```python
from build123d import *

# Parameters (mm, degrees)
SKETCH_W        = 19.05
SKETCH_H        = 9.525
PAD_DEPTH       = 215.9
SKETCH001_W     = 9.525
SKETCH001_H     = 2.38125
POCKET_DEPTH    = 215.901
SKETCH002_W     = 14.2875
SKETCH002_H     = 3.175
POCKET001_DEPTH = 215.901
SKETCH003_W     = 11.1125
SKETCH003_H     = 1.5875
POCKET002_DEPTH = 215.901


with BuildPart() as part:
    # Sketch → Pad (new body)
    with BuildSketch(Plane.XZ):
        Rectangle(SKETCH_W, SKETCH_H)
    extrude(amount=PAD_DEPTH)

    # Sketch001 (on Face6 of Pad) → Pocket (cut, through all)
    with BuildSketch(Plane.XZ.offset(215.9)):
        with Locations((0, 3.571875)):
            Rectangle(SKETCH001_W, SKETCH001_H)
    extrude(amount=-POCKET_DEPTH, mode=Mode.SUBTRACT)

    # Sketch002 (on Face5 of Pocket) → Pocket001 (cut, through all)
    with BuildSketch(Plane.XZ.offset(215.9)):
        with Locations((0, 0.79375)):
            Rectangle(SKETCH002_W, SKETCH002_H)
    extrude(amount=-POCKET001_DEPTH, mode=Mode.SUBTRACT)

    # Sketch003 (on Face5 of Pocket001) → Pocket002 (cut, through all)
    with BuildSketch(Plane.XZ.offset(215.9)):
        with Locations((0, -1.5875)):
            Rectangle(SKETCH003_W, SKETCH003_H)
    extrude(amount=-POCKET002_DEPTH, mode=Mode.SUBTRACT)


solid = part.part
```
Build history of the part. All positions in model axes, mm. Coordinates: 2 decimals unless noted, no trailing zeros. Order: outer loops, then holes, each group sorted by start corner. A loop starts at its lowest first (then second) coordinate and runs counter-clockwise, first axis right, second up. Notation, with made-up numbers: (-24.5, -12.75) -> (2.5, -12.75) arc R23 ccw to (2.5, 2.25) -> close; hole circle Ø9 at (87.25, 41). An arc over 180 degrees is marked (long way). Answer in a Markdown table with one row per item. Add a question column.
Q1. Wall check: line 1 along X through (y, z) = (-109.5, 0.75) (3 decimals); line 2 along Z through (x, y) = (5.5, -189.5); line 3 along Z through (x, y) = (-5.75, -182). Give the ranges that are in metal, low to high. Write a range as [from, to].
Q2. Drop a flat-ended pin along its axis: pin 1 (4 mm diameter, centred on x = 2.5, y = -59.5, fed in from +Z). Give the stop position or say it passes through.
Q3. Band-saw the part on A-A, the plane y = -69. List the corners of the cut face in (x, z) (1 decimal).
Q4. Mould opens along X. For faces 1 (the face through (-9.525, -106, 0)), 2 (the face through (0, 0, -3)), 3 (the face through (0, -109, -2.381)) say: +X half, -X half, draft (parallel to the pull), parting line (faces both ways), or undercut.
Q5. Band-saw the part on B-B, the plane x = 0.75. List the corners of the cut face in (y, z).
Answers follow:
| question | item | result |
|---|---|---|
| 1 | line 1 | [-9.525, -7.144], [7.144, 9.525] |
| 1 | line 2 | [-4.76, -2.38], [2.38, 4.76] |
| 1 | line 3 | [-4.76, -0.79], [2.38, 4.76] |
| 2 | pin 1 | z = -2.38 |
| 3 | outline | (-9.5, -4.8) -> (9.5, -4.8) -> (9.5, 4.8) -> (4.8, 4.8) -> (4.8, 2.4) -> (7.1, 2.4) -> (7.1, -0.8) -> (5.6, -0.8) -> (5.6, -2.4) -> (-5.6, -2.4) -> (-5.6, -0.8) -> (-7.1, -0.8) -> (-7.1, 2.4) -> (-4.8, 2.4) -> (-4.8, 4.8) -> (-9.5, 4.8) -> close |
| 4 | face 1 | -X half |
| 4 | face 2 | draft |
| 4 | face 3 | undercut |
| 5 | outline | (-215.9, -4.76) -> (0, -4.76) -> (0, -2.38) -> (-215.9, -2.38) -> close |
